Autodesk Inventor part; units mm, degrees
ref_plane "Work Plane2" through (0, 10, 0) normal (0, 1, 0) x (1, 0, 0)
ref_plane "YZ Plane" through (0, 0, 0) normal (1, 0, 0) x (0, 1, 0)
ref_plane "XZ Plane" through (0, 0, 0) normal (0, 1, 0) x (-1, 0, 0)
sketch "Sketch1" plane through (0, 0, 0) normal (0, 1, 0) x (-1, 0, 0)
  circle A0 centre (0, 0) radius 57.25
  circle A1 centre (0, 0) radius 52.25
  circle A2 centre (0, 0) radius 50.4125
  circle A3 centre (0, 0) radius 9.5
  dimension "Absolute_Diameter" = 114.5
  dimension "Diameter_No_Outer_Lip" = 104.5
  dimension "Inner_Cylinder_Diameter" = 100.825
  dimension "Lip_Diameter" = 19
extrude "Extrusion1" add sketch "Sketch1" along normal blind 5 contours A0
extrude "Extrusion2" add sketch "Sketch1" along normal blind 75 contours A1
sketch "Sketch2" plane through (0, 75, 0) normal (0, 1, 0) x (1, 0, 0)
  circle A0 centre (0, 0) radius 52.25
  circle A1 centre (0, 0) radius 45.875
  dimension "Lip_Diameter_Out" = 104.5
  dimension "Inner_Lip_Diameter" = 91.75
extrude "Extrusion7" add sketch "Sketch2" against normal blind 5
ref_plane "Work Plane2" through (0, 10, 0) normal (0, 1, 0) x (1, 0, 0)
sketch "Sketch3" plane through (0, 10, 0) normal (0, 1, 0) x (1, 0, 0)
  circle A0 centre (0, 0) radius 127.5
  circle A1 centre (0, 127.5) radius 2.75
  circle A2 centre (-74.9426, 103.1497) radius 2.75
  circle A3 centre (-121.2597, 39.3997) radius 2.75
  circle A4 centre (-121.2597, -39.3997) radius 2.75
  circle A5 centre (-74.9426, -103.1497) radius 2.75
  circle A6 centre (0, -127.5) radius 2.75
  circle A7 centre (74.9426, -103.1497) radius 2.75
  circle A8 centre (121.2597, -39.3997) radius 2.75
  circle A9 centre (121.2597, 39.3997) radius 2.75
  circle A10 centre (74.9426, 103.1497) radius 2.75
  dimension "d27" = 255
  dimension "d229" = 5.5
  dimension "d232" = 360
extrude "Extrusion8" [suppressed]
sketch "Sketch24" plane through (0, 0, 0) normal (0, -1, 0) x (1, 0, 0)
  circle A0 centre (0, 0) radius 112.0375
  arc A1 (-85.157, -104.7535) -> (32.5, -131.0296) centre (0, 0) ccw
  circle A2 centre (0, 0) radius 133
  line L0 (-32.5, -70.125) -> (32.5, -70.125)
  line L1 (32.5, -70.125) -> (32.5, -160.125)
  line L2 (32.5, -160.125) -> (-32.5, -160.125)
  line L3 (-32.5, -160.125) -> (-32.5, -70.125)
  line L4 (-31, -158.625) -> (31, -158.625)
  line L5 (31, -158.625) -> (31, -71.625)
  line L6 (31, -71.625) -> (-31, -71.625)
  line L7 (-31, -71.625) -> (-31, -158.625)
  line L8 (-85.157, -65.125) -> (-46.3, -65.125)
  line L9 (-46.3, -65.125) -> (-46.3, -151.2985)
  line L10 (-46.3, -151.2985) -> (-85.157, -151.2985)
  line L11 (-85.157, -151.2985) -> (-85.157, -65.125)
  arc A3 (32.5, -131.0296) -> (-85.157, -104.7535) centre (0, 0) ccw
  line L12 (0, -71.625) -> (0, -158.625)
  line L13 (-83.157, -149.2985) -> (-48.3, -149.2985)
  line L14 (-48.3, -149.2985) -> (-48.3, -67.125)
  line L15 (-48.3, -67.125) -> (-83.157, -67.125)
  line L16 (-83.157, -67.125) -> (-83.157, -149.2985)
  line L17 (85.157, -65.125) -> (46.3, -65.125)
  line L18 (46.3, -65.125) -> (46.3, -151.2985)
  line L19 (46.3, -151.2985) -> (85.157, -151.2985)
  line L20 (85.157, -151.2985) -> (85.157, -65.125)
  line L21 (83.157, -149.2985) -> (48.3, -149.2985)
  line L22 (48.3, -149.2985) -> (48.3, -67.125)
  line L23 (48.3, -67.125) -> (83.157, -67.125)
  line L24 (83.157, -67.125) -> (83.157, -149.2985)
  circle A4 centre (0, 0) radius 120
  point P0 (0, -135)
  point P1 (48.3, -126.0639)
  point P2 (83.157, -106.3481)
  point P3 (-31, -131.3925)
  point P4 (31, -131.3925)
  point P5 (-83.157, -106.3481)
  point P6 (-48.3, -126.0639)
  point P7 (46.3, -126.8121)
  point P8 (85.157, -104.7535)
  point P9 (-32.5, -131.0296)
  point P10 (-46.3, -126.8121)
  point P11 (48.3, -109.8504)
  point P12 (48.3, -101.0916)
  point P13 (31, -107.6634)
  point P14 (31, -115.9267)
  point P15 (-48.3, -109.8504)
  point P16 (-31, -115.9267)
  point P17 (-31, -107.6634)
  point P18 (-48.3, -101.0916)
  dimension "d234" = 2
  dimension "d235" = 65
  dimension "d237" = 1.5
  dimension "d238" = 11.113
  dimension "d240" = 20.9625
  dimension "d241" = 270
  dimension "d242" = 90
  dimension "d243" = 153.238
  dimension "d244" = 228.338
  dimension "d247" = 2
  dimension "d248" = 129.75
  dimension "d253" = 240
extrude "Extrusion30" [suppressed]
extrude "Extrusion31" [suppressed]
extrude "Extrusion32" [suppressed]
fillet "Fillet14" [suppressed]
fillet "Fillet15" [suppressed]
fillet "Fillet16" [suppressed]
fillet "Fillet17" [suppressed]
fillet "Fillet18" [suppressed]
sketch "Sketch25" plane through (0, 70, 0) normal (0, -1, 0) x (1, 0, 0)
  circle A0 centre (0, 0) radius 112.0375
  circle A1 centre (0, 0) radius 115
extrude "Extrusion33" [suppressed]
properties part number "Cylinder  Segment - 10"
For this review, take the finished solid that the model builds, in its own axes (mm). A direction names the side the tool comes from. Give positions to 0.01 mm unless a question says otherwise; leave off trailing zeros. One line per item, written item: value. Start each with the question number.
Q1. Draft analysis for pull direction Z (two halves, no side actions). For faces 4 (the face through (0, 0, -51)), 5 (the face through (-28.089, 39.51, -44.057)), 6 (the face through (-5.972, 72.535, -45.485)), state which applies: released by +Z, released by -Z, zero draft, split by the parting line, or undercut.
Q2. Machinability: for faces 1 (the face through (11, 70, 45)), 2 (the face through (-51, 5, 13)), 3 (the face through (12.41, 2.46, 55.89)), which of the approach directions +Z, -Z, +X, -X, +Y, -Y give a long, thin tool a straight path to every point of the face, cutting with its end or side? Answer none if there is none.
Q3. For L1, parallel to Z at x = 0, y = 18; L2, parallel to Z at x = 0, y = 72.1 (3 decimals); L3, parallel to X at y = 67, z = -17, list the stretches that pass through material, from the lowest coordinate up.
Q4. Clearance check with flat-ended pins moving along their axes: pin 1 Ø4 at (y, z) = (42, 34) entering from +X; pin 2 Ø4 at (y, z) = (8, 1) entering from +X; pin 3 Ø10 at (x, y) = (28, 44) entering from +Z. State where each tip first meets the part, or that it passes through.
Reply:
1. face 4: zero draft
1. face 5: split by the parting line
1. face 6: undercut
2. face 1: -Y
2. face 2: +Y
2. face 3: +Y, -Y
3. L1: -52.25 to -50.41, 50.41 to 52.25
3. L2: -52.25 to -45.875, 45.875 to 52.25
3. L3: -49.41 to -47.46, 47.46 to 49.41
4. pin 1: x = 41.3
4. pin 2: x = 52.25
4. pin 3: z = 46.92
